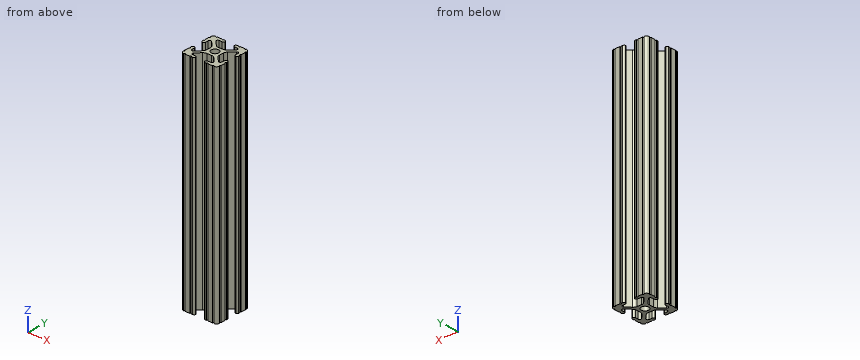
```python
from build123d import *

# Parameters (mm, degrees)
SKETCH1_R           = 2.6035
BOSS_EXTRUDE1_DEPTH = 304.8
SKETCH2_R           = 37.713648337
CUT_EXTRUDE1_DEPTH  = 203.2
SKETCH4_R           = 34.529117014
CUT_EXTRUDE3_DEPTH  = 254
SKETCH5_R           = 0.254
CUT_EXTRUDE4_DEPTH  = 254


with BuildPart() as part:
    # Sketch1 → Boss-Extrude1 (new, symmetric)
    with BuildSketch(Plane.XY):
        with BuildLine():
            Line((-7.179650497, -8.645192506), (-3.952270251, -5.423690499))
            ThreePointArc((-3.952270251, -5.423690499), (-2.922936451, -4.736929036), (-1.709253557, -4.4958))
            Line((-1.709253557, -4.4958), (1.709253557, -4.4958))
            ThreePointArc((1.709253557, -4.4958), (2.922936451, -4.736929036), (3.952270251, -5.423690499))
            Line((3.952270251, -5.423690499), (7.179650497, -8.645192506))
            ThreePointArc((7.179650497, -8.645192506), (7.41473083, -9.822813117), (6.416408329, -10.4902))
            Line((6.416408329, -10.4902), (4.287512407, -10.4902))
            ThreePointArc((4.287512407, -10.4902), (3.54574862, -10.79744862), (3.2385, -11.539212407))
            Line((3.2385, -11.539212407), (3.2385, -11.650987593))
            ThreePointArc((3.2385, -11.650987593), (3.54574862, -12.39275138), (4.287512407, -12.7))
            Line((4.287512407, -12.7), (5.317126718, -12.7))
            ThreePointArc((5.317126718, -12.7), (5.825126718, -12.192), (6.333126718, -12.7))
            Line((6.333126718, -12.7), (9.550443118, -12.7))
            ThreePointArc((9.550443118, -12.7), (10.058366869, -12.192000006), (10.566443095, -12.699847501))
            ThreePointArc((10.566443095, -12.699847501), (12.082537762, -12.08250727), (12.699846982, -10.566399977))
            ThreePointArc((12.699846982, -10.566399977), (12.192000006, -10.058323491), (12.7, -9.5504))
            Line((12.7, -9.5504), (12.7, -6.3330836))
            ThreePointArc((12.7, -6.3330836), (12.192, -5.8250836), (12.7, -5.3170836))
            Line((12.7, -5.3170836), (12.7, -4.287469289))
            ThreePointArc((12.7, -4.287469289), (12.39275138, -3.545705502), (11.650987593, -3.238456882))
            Line((11.650987593, -3.238456882), (11.539212407, -3.238456882))
            ThreePointArc((11.539212407, -3.238456882), (10.79744862, -3.545705502), (10.4902, -4.287469289))
            Line((10.4902, -4.287469289), (10.4902, -6.402089023))
            ThreePointArc((10.4902, -6.402089023), (9.856505071, -7.351067942), (8.737131347, -7.129408934))
            Line((8.737131347, -7.129408934), (5.441005833, -3.840816462))
            ThreePointArc((5.441005833, -3.840816462), (4.750877967, -2.809883091), (4.5085, -1.593185507))
            Line((4.5085, -1.593185507), (4.5085, 1.593185507))
            ThreePointArc((4.5085, 1.593185507), (4.750877967, 2.809883091), (5.441005833, 3.840816462))
            Line((5.441005833, 3.840816462), (8.737131347, 7.129408934))
            ThreePointArc((8.737131347, 7.129408934), (9.856505071, 7.351067942), (10.4902, 6.402089023))
            Line((10.4902, 6.402089023), (10.4902, 4.287469289))
            ThreePointArc((10.4902, 4.287469289), (10.79744862, 3.545705502), (11.539212407, 3.238456882))
            Line((11.539212407, 3.238456882), (11.650987593, 3.238456882))
            ThreePointArc((11.650987593, 3.238456882), (12.39275138, 3.545705502), (12.7, 4.287469289))
            Line((12.7, 4.287469289), (12.7, 5.3170836))
            ThreePointArc((12.7, 5.3170836), (12.192, 5.8250836), (12.7, 6.3330836))
            Line((12.7, 6.3330836), (12.7, 9.5504))
            ThreePointArc((12.7, 9.5504), (12.192000006, 10.058323491), (12.699846982, 10.566399977))
            ThreePointArc((12.699846982, 10.566399977), (12.082537762, 12.08250727), (10.566443095, 12.699847501))
            ThreePointArc((10.566443095, 12.699847501), (10.058366869, 12.192000006), (9.550443118, 12.7))
            Line((9.550443118, 12.7), (6.333126718, 12.7))
            ThreePointArc((6.333126718, 12.7), (5.825126718, 12.192), (5.317126718, 12.7))
            Line((5.317126718, 12.7), (4.287512407, 12.7))
            ThreePointArc((4.287512407, 12.7), (3.54574862, 12.39275138), (3.2385, 11.650987593))
            Line((3.2385, 11.650987593), (3.2385, 11.539212407))
            ThreePointArc((3.2385, 11.539212407), (3.54574862, 10.79744862), (4.287512407, 10.4902))
            Line((4.287512407, 10.4902), (6.476788598, 10.4902))
            ThreePointArc((6.476788598, 10.4902), (7.432222385, 9.85140422), (7.207036008, 8.724370562))
            Line((7.207036008, 8.724370562), (3.898272566, 5.423169045))
            ThreePointArc((3.898272566, 5.423169045), (2.869120213, 4.736787962), (1.655778399, 4.4958))
            Line((1.655778399, 4.4958), (-1.655778399, 4.4958))
            ThreePointArc((-1.655778399, 4.4958), (-2.869120213, 4.736787962), (-3.898272566, 5.423169045))
            Line((-3.898272566, 5.423169045), (-7.207036008, 8.724370562))
            ThreePointArc((-7.207036008, 8.724370562), (-7.432222385, 9.85140422), (-6.476788598, 10.4902))
            Line((-6.476788598, 10.4902), (-4.287512407, 10.4902))
            ThreePointArc((-4.287512407, 10.4902), (-3.54574862, 10.79744862), (-3.2385, 11.539212407))
            Line((-3.2385, 11.539212407), (-3.2385, 11.650987593))
            ThreePointArc((-3.2385, 11.650987593), (-3.54574862, 12.39275138), (-4.287512407, 12.7))
            Line((-4.287512407, 12.7), (-5.317126718, 12.7))
            ThreePointArc((-5.317126718, 12.7), (-5.825126718, 12.192), (-6.333126718, 12.7))
            Line((-6.333126718, 12.7), (-9.550443118, 12.7))
            ThreePointArc((-9.550443118, 12.7), (-10.058366869, 12.192000006), (-10.566443095, 12.699847501))
            ThreePointArc((-10.566443095, 12.699847501), (-12.082537762, 12.08250727), (-12.699846982, 10.566399977))
            ThreePointArc((-12.699846982, 10.566399977), (-12.192000006, 10.058323491), (-12.7, 9.5504))
            Line((-12.7, 9.5504), (-12.7, 6.3330836))
            ThreePointArc((-12.7, 6.3330836), (-12.192, 5.8250836), (-12.7, 5.3170836))
            Line((-12.7, 5.3170836), (-12.7, 4.287469289))
            ThreePointArc((-12.7, 4.287469289), (-12.39275138, 3.545705502), (-11.650987593, 3.238456882))
            Line((-11.650987593, 3.238456882), (-11.539212407, 3.238456882))
            ThreePointArc((-11.539212407, 3.238456882), (-10.79744862, 3.545705502), (-10.4902, 4.287469289))
            Line((-10.4902, 4.287469289), (-10.4902, 6.402089023))
            ThreePointArc((-10.4902, 6.402089023), (-9.856505071, 7.351067942), (-8.737131347, 7.129408934))
            Line((-8.737131347, 7.129408934), (-5.441005833, 3.840816462))
            ThreePointArc((-5.441005833, 3.840816462), (-4.750877967, 2.809883091), (-4.5085, 1.593185507))
            Line((-4.5085, 1.593185507), (-4.5085, -1.593185507))
            ThreePointArc((-4.5085, -1.593185507), (-4.750877967, -2.809883091), (-5.441005833, -3.840816462))
            Line((-5.441005833, -3.840816462), (-8.737131347, -7.129408934))
            ThreePointArc((-8.737131347, -7.129408934), (-9.856505071, -7.351067942), (-10.4902, -6.402089023))
            Line((-10.4902, -6.402089023), (-10.4902, -4.287469289))
            ThreePointArc((-10.4902, -4.287469289), (-10.79744862, -3.545705502), (-11.539212407, -3.238456882))
            Line((-11.539212407, -3.238456882), (-11.650987593, -3.238456882))
            ThreePointArc((-11.650987593, -3.238456882), (-12.39275138, -3.545705502), (-12.7, -4.287469289))
            Line((-12.7, -4.287469289), (-12.7, -5.3170836))
            ThreePointArc((-12.7, -5.3170836), (-12.192, -5.8250836), (-12.7, -6.3330836))
            Line((-12.7, -6.3330836), (-12.7, -9.5504))
            ThreePointArc((-12.7, -9.5504), (-12.192000006, -10.058323491), (-12.699846982, -10.566399977))
            ThreePointArc((-12.699846982, -10.566399977), (-12.082537762, -12.08250727), (-10.566443095, -12.699847501))
            ThreePointArc((-10.566443095, -12.699847501), (-10.058366869, -12.192000006), (-9.550443118, -12.7))
            Line((-9.550443118, -12.7), (-6.333126718, -12.7))
            ThreePointArc((-6.333126718, -12.7), (-5.825126718, -12.192), (-5.317126718, -12.7))
            Line((-5.317126718, -12.7), (-4.287512407, -12.7))
            ThreePointArc((-4.287512407, -12.7), (-3.54574862, -12.39275138), (-3.2385, -11.650987593))
            Line((-3.2385, -11.650987593), (-3.2385, -11.539212407))
            ThreePointArc((-3.2385, -11.539212407), (-3.54574862, -10.79744862), (-4.287512407, -10.4902))
            Line((-4.287512407, -10.4902), (-6.416408329, -10.4902))
            ThreePointArc((-6.416408329, -10.4902), (-7.41473083, -9.822813117), (-7.179650497, -8.645192506))
        make_face()
        Circle(SKETCH1_R, mode=Mode.SUBTRACT)
    extrude(amount=BOSS_EXTRUDE1_DEPTH, both=True)

    # Sketch2 → Cut-Extrude1 (cut)
    with BuildSketch(Plane.XY.offset(304.8)):
        Circle(SKETCH2_R)
    extrude(amount=-CUT_EXTRUDE1_DEPTH, mode=Mode.SUBTRACT)

    # Sketch4 → Cut-Extrude3 (cut)
    with BuildSketch(Plane.XY.offset(101.6)):
        Circle(SKETCH4_R)
    extrude(amount=-CUT_EXTRUDE3_DEPTH, mode=Mode.SUBTRACT)

    # Sketch5 → Cut-Extrude4 (cut)
    with BuildSketch(Plane(origin=(4.5085, 0, 0), x_dir=(0, 0, -1), z_dir=(1, 0, 0))):
        with Locations((228.6, 0)):
            Circle(SKETCH5_R)
    extrude(amount=-CUT_EXTRUDE4_DEPTH, mode=Mode.SUBTRACT)


solid = part.part
```
Here's how the part is built. I have some questions about the finished solid (model axes, mm). Give positions to 0.01 mm unless a question says otherwise; leave off trailing zeros. Loops run counter-clockwise (first coordinate to the right, second up) from the corner with the lowest first, then second, coordinate; pieces in that order, holes last. Notation, with made-up numbers: M 66.5,16.25 L 90.5,16.25 A12 cw 90.5,32.25 Z; hole C 57,51.25 d11. An arc over 180 degrees is marked long. Use one line per item in the form item = value. Start each with the question number.
Q1. Will these pins go through, and if not, where does the flat tip stop? pin 1 Ø4 at (x, z) = (0.5, -194) entering from -Y; pin 2 Ø2.5 at (y, z) = (0.5, -250) entering from -X; pin 3 Ø3 at (y, z) = (-2.5, -226.5) entering from +X.
Q2. If we section it at A-A (x = 0): Write out the boundary of the cut face in (y, z), then the cut area to 3 significant figures.
Q3. I need wall thicknesses on line 1 along Y through (x, z) = (0, -209.5); line 2 along Y through (x, z) = (-2, -201); line 3 along Y through (x, z) = (-3.7, -228.6). Which ranges of each line are inside material? Lowest first, please.
Taken from the geometry:
q1.pin_1 = -4.6
q1.pin_2 = -4.51
q1.pin_3 = 12.66
q2.outline = M -4.5,-304.8 L -2.6,-304.8 L -2.6,-152.4 L -4.5,-152.4 Z; M 2.6,-304.8 L 4.5,-304.8 L 4.5,-152.4 L 2.6,-152.4 Z
q2.area = 577 mm^2
q3.line_1 = -4.5 to -2.6, 2.6 to 4.5
q3.line_2 = -4.51 to -1.67, 1.67 to 4.51
q3.line_3 = -12.52 to -10.67, -5.2 to -0.25, 0.25 to 5.24, 10.67 to 12.52
